Can you work these out from the model? Positions are in its coordinate system, mm. Coordinates: 2 decimals unless noted, no trailing zeros. Loops run counter-clockwise (first coordinate to the right, second up) from the corner with the lowest first, then second, coordinate; pieces in that order, holes last. Notation, with made-up numbers: (-0.5, -39.75) -> (40.5, -39.75) arc R21 ccw to (40.5, -30.75) -> close; hole circle Ø4 at (-34, 25). An arc over 180 degrees is marked (long way). Use one line per item in the form item = value. Start each with the question number.
(1) Imagine slicing it at C-C (x = -4.75). List the corners of the cut face in (y, z) for me.
(2) Imagine slicing it at D-D (y = -7). List the corners of the cut face in (x, z) for me, plus the area to 3 significant figures.
(3) Imagine slicing it at A-A (y = 0). List the corners of the cut face in (x, z) for me.
(4) I need wall thicknesses on line 1 (Y direction, x = 1.25, z = 165.5); line 2 (X direction, y = -8.5, z = 10.5); line 3 (X direction, y = -0.5, z = 85). Which ranges of each line are inside material? Lowest first, please. Write a range as [from, to].
(5) Imagine slicing it at B-B (z = 21.5). List the corners of the cut face in (x, y) for me (1 decimal).
(6) I'm going to push flat-ended pins straight in: pin 1 (6 mm diameter, centred on x = -4, z = 146.5, fed in from -Y); pin 2 (3 mm diameter, centred on y = 6.5, z = 99.5, fed in from +X); pin 3 (1 mm diameter, centred on x = 2.5, z = 54.5, fed in from -Y). Where does each tip first touch, or does it pass through?
```python
from build123d import *

# Parameters (mm, degrees)
SKETCH1_R           = 9.8425
BOSS_EXTRUDE1_DEPTH = 190.5
BOSS_EXTRUDE6_DEPTH = 10.16


with BuildPart() as part:
    # Sketch1 → Boss-Extrude1 (new body)
    with BuildSketch(Plane.XY):
        Circle(SKETCH1_R)
    extrude(amount=BOSS_EXTRUDE1_DEPTH)

    # Sketch6 → Boss-Extrude6 (add)
    with BuildSketch(Plane(origin=(0, 0, 0), x_dir=(0, 0, -1), z_dir=(1, 0, 0))):
        with BuildLine():
            Line((-1.301661294, 2.396009349), (-1.301661294, -3.953990651))
            ThreePointArc((-1.301661294, -3.953990651), (-2.161224479, -4.813553836), (-3.020787664, -3.953990651))
            Line((-3.020787664, -3.953990651), (-3.020787664, 2.396009349))
            ThreePointArc((-3.020787664, 2.396009349), (-2.161224479, 3.255572534), (-1.301661294, 2.396009349))
        make_face()
    extrude(amount=BOSS_EXTRUDE6_DEPTH)


solid = part.part
```
Worked out:
q1.outline = (-8.62, 0) -> (8.62, 0) -> (8.62, 190.5) -> (-8.62, 190.5) -> close
q2.outline = (-6.92, 0) -> (6.92, 0) -> (6.92, 190.5) -> (-6.92, 190.5) -> close
q2.area = 2,640 mm2
q3.outline = (-9.84, 0) -> (9.84, 0) -> (9.84, 1.3) -> (10.16, 1.3) -> (10.16, 3.02) -> (9.84, 3.02) -> (9.84, 190.5) -> (-9.84, 190.5) -> close
q4.line_1 = [-9.76, 9.76]
q4.line_2 = [-4.96, 4.96]
q4.line_3 = [-9.83, 9.83]
q5.outline = circle Ø19.7 at (0, 0)
q6.pin_1 = -9.79
q6.pin_2 = 8.48
q6.pin_3 = -9.64
